Source: CAD feature listing. Evaluate the final solid. Frame: model axes, mm. Give positions to 0.01 mm unless a question says otherwise; leave off trailing zeros. Loops run counter-clockwise (first coordinate to the right, second up) from the corner with the lowest first, then second, coordinate; pieces in that order, holes last. Notation, with made-up numbers: (88, 41.25) - (122, 41.25) arc R19 cw to (122, 76.25) - close; hole circle Ø1 at (-33, -24.5). An arc over 180 degrees is marked (long way). Write each question's results on one line, items separated by ' | '. Start each with the question number.
(1) Cut plane C-C on y = 300.5. Return the cut outline in (x, z).
(2) Contact query for flat-ended pins moving along their axis: pin 1 (5 mm diameter, centred on x = 6, z = 364.5, fed in from -Y); pin 2 (6 mm diameter, centred on x = 7, z = 173.5, fed in from -Y); pin 3 (4 mm diameter, centred on x = 7, y = 51.5, fed in from -Z). Output: stop coordinate, or through.
(3) Cut plane B-B on z = 63. Return the cut outline in (x, y).
(4) Cut plane A-A on x = 6. Return the cut outline in (y, z).
(5) Material intervals for line 1 along Y through (x, z) = (0.5, 126); line 2 along Y through (x, z) = (4.25, 374); line 3 along Z through (x, y) = (3.5, 124), sorted ascending. Write a range as [from, to].
from build123d import *

# Parameters (mm, degrees)
F1_DEPTH = 12.7


with BuildPart() as f1:
    # F0 (on Right) → F1 (new body)
    with BuildSketch(Plane.YZ):
        Polygon((5.305482, 480.825944), (-8.301662, -27.174056), (398.098338, -24.906198), (361.476894, 38.696464), (152.353483, 401.893668), (106.905482, 480.825944), align=None)
        Polygon((152.353483, 401.893668), (361.476894, 38.696464), (372.48287, 45.033538), (334.460432, 111.069393), (315.449213, 144.08732), (277.426774, 210.123176), (258.415555, 243.141103), (220.393116, 309.176958), (201.381897, 342.194886), (163.359459, 408.230741), align=None)
    extrude(amount=F1_DEPTH)


solid = f1.part
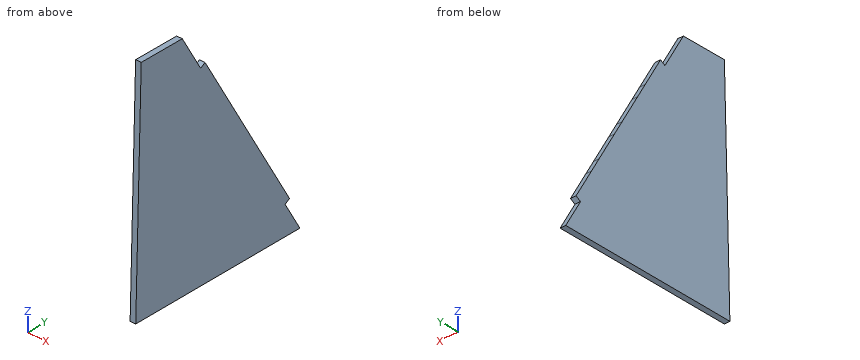
Ans:
1) outline: (0, -25.45) - (12.7, -25.45) - (12.7, 170.05) - (0, 170.05) - close
2) pin 1: y = 2.12 | pin 2: y = -3.01 | pin 3: z = -26.85
3) outline: (0, -5.89) - (12.7, -5.89) - (12.7, 362.14) - (0, 362.14) - close
4) outline: (-8.3, -27.17) - (398.1, -24.91) - (361.48, 38.7) - (372.48, 45.03) - (163.36, 408.23) - (152.35, 401.89) - (106.91, 480.83) - (5.31, 480.83) - close
5) line 1: [-4.2, 325.86] | line 2: [2.44, 183.07] | line 3: [-26.44, 451.14]
